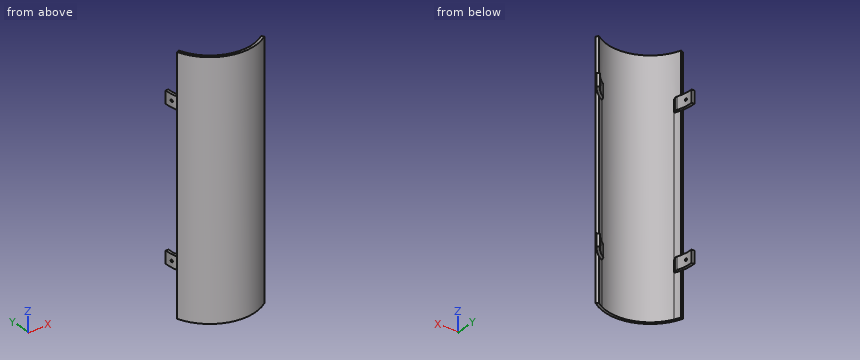
```python
from build123d import *

# Parameters (mm, degrees)
EXTRUDE_1_DEPTH     = 150
EXTRUDE_START       = -247.5
EXTRUDE_2_DEPTH     = 247.5
CUT_EXTRUDE_START   = -52.5
SKETCH_3_R          = 51.8
CUT_EXTRUDE_1_DEPTH = 52.5
SKETCH_4_R          = 51.8
CUT_EXTRUDE_2_DEPTH = 82.5
SKETCH_6_R          = 1.5
CUT_EXTRUDE_3_DEPTH = 165
SKETCH_7_R          = 1.5
CUT_EXTRUDE_4_DEPTH = 165


with BuildPart() as part:
    # 草图1 → 凸台-拉伸1 (new, symmetric)
    with BuildSketch(Plane.XY):
        with BuildLine():
            Line((-52.413174316, -16.669107897), (-49.363680538, -15.699268892))
            ThreePointArc((-49.363680538, -15.699268892), (-16.314268086, -49.163855187), (30.185108172, -42.096309157))
            Line((30.185108172, -42.096309157), (32.049825279, -44.696853352))
            ThreePointArc((32.049825279, -44.696853352), (-17.322099319, -52.201004542), (-52.413174316, -16.669107897))
        make_face()
    extrude(amount=EXTRUDE_1_DEPTH, both=True)

    # 草图2 → 凸台-拉伸2 (add)
    with BuildSketch(Plane(origin=(0, 0, -150), x_dir=(-1, 0, 0), z_dir=(0, 0, -1)).offset(EXTRUDE_START)):
        with BuildLine():
            Line((-24.924043095, -42.002946324), (-23.507517235, -46.158819671))
            ThreePointArc((-23.507517235, -46.158819671), (-34.198599667, -38.906243468), (-42.762509098, -29.233676054))
            Line((-42.762509098, -29.233676054), (-40.120809695, -27.427734676))
            ThreePointArc((-40.120809695, -27.427734676), (-33.774000748, -34.946772003), (-26.042778843, -41.033323898))
            ThreePointArc((-26.042778843, -41.033323898), (-25.447325167, -41.476499857), (-24.924043095, -42.002946324))
        make_face()
        with BuildLine():
            Line((48.558861257, 1.99924822), (51.756152533, 2.130885963))
            ThreePointArc((51.756152533, 2.130885963), (50.673816706, -10.742639362), (46.439539695, -22.947966205))
            Line((46.439539695, -22.947966205), (45.090508335, -18.769695848))
            ThreePointArc((45.090508335, -18.769695848), (45.195249795, -18.034849445), (45.40762753, -17.323607076))
            ThreePointArc((45.40762753, -17.323607076), (47.966326083, -7.822503569), (48.558861257, 1.99924822))
        make_face()
    extrude(amount=EXTRUDE_2_DEPTH)

    # 草图3 → 切除-拉伸1 (cut)
    with BuildSketch(Plane(origin=(0, 0, -150), x_dir=(-1, 0, 0), z_dir=(0, 0, -1)).offset(CUT_EXTRUDE_START)):
        Circle(SKETCH_3_R)
    extrude(amount=CUT_EXTRUDE_1_DEPTH, mode=Mode.SUBTRACT)

    # 草图4 → 切除-拉伸2 (cut, symmetric)
    with BuildSketch(Plane.XY):
        Circle(SKETCH_4_R)
    extrude(amount=CUT_EXTRUDE_2_DEPTH, both=True, mode=Mode.SUBTRACT)

    # 草图6 → 切除-拉伸3 (cut)
    with BuildSketch(Plane(origin=(0, 0, 0), x_dir=(-0.6991347993064156, -0.7149898827247683, 0), z_dir=(0.7149898827247683, -0.6991347993064156, 0))):
        with Locations((0, 90)):
            Circle(SKETCH_6_R)
        with Locations((0, -90)):
            Circle(SKETCH_6_R)
    extrude(amount=CUT_EXTRUDE_3_DEPTH, mode=Mode.SUBTRACT)

    # 草图7 → 切除-拉伸4 (cut)
    with BuildSketch(Plane(origin=(0, 0, 0), x_dir=(0.13298935431462466, -0.991117466115384, 0), z_dir=(0.991117466115384, 0.13298935431462466, 0))):
        with Locations(Location((0, 90, 0), (0, 0, 180))):
            Circle(SKETCH_7_R)
        with Locations(Location((0, -90, 0), (0, 0, 180))):
            Circle(SKETCH_7_R)
    extrude(amount=-CUT_EXTRUDE_4_DEPTH, mode=Mode.SUBTRACT)


solid = part.part
```
Read the model definition and answer for the solid it produces. Units are mm, in the model's axes. Round coordinates to 2 decimals unless told otherwise and drop trailing zeros. Write each loop counter-clockwise with the first axis right and the second up, starting at its lowest first coordinate (ties: lowest second). Pieces come first, ordered by that corner, then holes. Notation, with made-up numbers: (55, -15) -> (61, -15) arc R25 cw to (61, -1) -> close; hole circle Ø4 at (16, 84). An arc over 180 degrees is marked (long way). Answer in a Markdown table with one row per item. Add a question column.
1) Find section D-D, the plane x = 1.5. Determine the outline of the cut face in (y, z).
2) Find section A-A, the plane y = -12.5. Determine the outline of the cut face in (x, z), and give its area (3 significant figures).
3) Consider line 1 (X direction, y = -44, z = 131); line 2 (X direction, y = -43.5, z = -40); line 3 (Y direction, x = 2, z = 11.5). Determine where each line is inside the solid, lowest interval first.
4) Find section B-B, the plane z = 14. Determine the outline of the cut face in (x, y).
5) Find section C-C, the plane x = 13.5. Determine the outline of the cut face in (y, z).
6) Given P1, Ø5.5, axis at x = -49.5, y = -8.5, coming from the +Z side; P2, Ø2, axis at x = -49.5, y = -6, coming from the -Z side; P3, Ø20.5, axis at x = 37.5, y = -38, coming from the +Z side; P4, Ø3, axis at y = -40, z = -111, coming from the +X side, each flat-ended and moving along its own axis, determine where each tip first touches the part or whether it passes through.
Findings below:
| question | item | result |
|---|---|---|
| 1 | outline | (-54.98, -150) -> (-51.78, -150) -> (-51.78, 150) -> (-54.98, 150) -> close |
| 2 | outline | (-50.27, -97.5) -> (-46.96, -97.5) -> (-46.96, -82.5) -> (-50.27, -82.5) -> close; (-50.27, 82.5) -> (-46.96, 82.5) -> (-46.96, 97.5) -> (-50.27, 97.5) -> close |
| 2 | area | 99.1 mm² |
| 3 | line 1 | -33 to -27.34, 27.34 to 31.55 |
| 3 | line 2 | -33.66 to -28.12, 28.12 to 31.19 |
| 3 | line 3 | -54.96 to -51.76 |
| 4 | outline | (-52.41, -16.67) arc R55 ccw to (32.05, -44.7) -> (30.19, -42.1) arc R51.8 cw to (-49.36, -15.7) -> close |
| 5 | outline | (-53.32, -150) -> (-50.01, -150) -> (-50.01, 150) -> (-53.32, 150) -> close |
| 6 | P1 | z = 97.5 |
| 6 | P2 | z = -97.5 |
| 6 | P3 | z = 150 |
| 6 | P4 | x = -31 |
